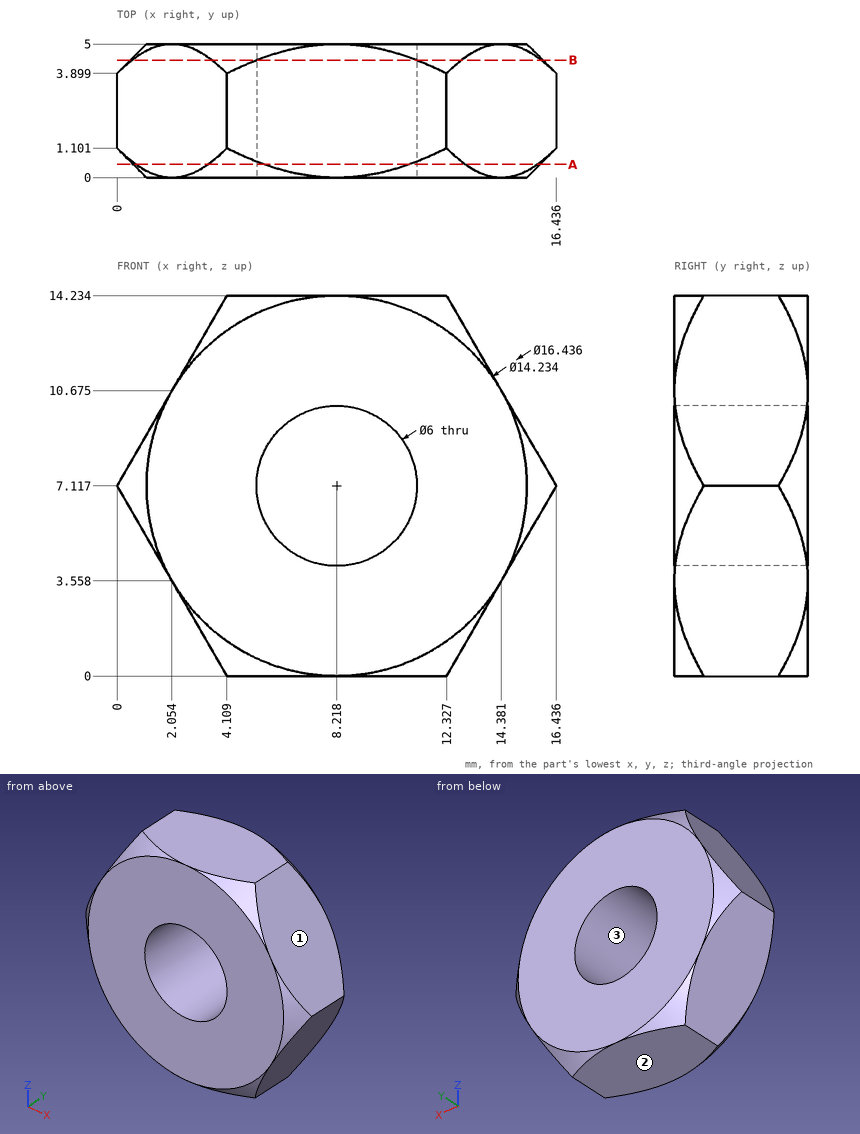
The figure shows three views and two pictorial views of one solid part (mm, origin at its lowest corner). Answer the questions. Give positions to 0.01 mm unless a question says otherwise; leave off trailing zeros. Order: outer loops, then holes, each group sorted by start corner. A loop starts at its lowest first (then second) coordinate and runs counter-clockwise, first axis right, second up. Notation, with made-up numbers: (36.5, 12) -> (53.5, 12) arc R11 ccw to (53.5, 27) -> close; hole circle Ø9 at (-17, 71.5). An arc over 180 degrees is marked (long way). Answer as a JSON object with one key per item and string values. Group by question number.
Item 1: Flat-ended cylindrical pins translate along their axes: pin 1 (1 mm diameter, centred on y = 4, z = 6, fed in from -X) (1 decimal); pin 2 (1.5 mm diameter, centred on y = 1, z = 12, fed in from -X) (1 decimal). Find the tip coordinate at first contact, or state that the pin passes through.
Item 2: Consider L1, parallel to X at y = 4.35, z = 8.25 (1 decimal); L2, parallel to Z at x = 6.75, y = 0.7 (1 decimal); L3, parallel to X at y = 2.35, z = 9.5 (1 decimal). Determine where each line is inside the solid, lowest interval first. Write a range as from..to.
Item 3: Determine the mould class of the marked faces 1, 2 and 3 for opening direction Z: pulls with the +Z half, pulls with the -Z half, needs draft (parallel to the pull), parting line crosses it, or undercut.
Item 4: The part is cut by section A-A on y = 0.5. Write down the section's boundary in (x, z) (1 decimal).
Item 5: The part is cut by section B-B on y = 4.4. Write down the section's boundary in (x, z) (1 decimal).
Result set:
{
 "1": {"pin 1": "x = 0.4", "pin 2": "x = 2.4"},
 "2": {"L1": "0.7..5.4, 11..15.8", "L2": "0..4.5, 9.7..14.2", "L3": "1.4..6.4, 10..15.1"},
 "3": {"face 1": "pulls with the +Z half", "face 2": "pulls with the -Z half", "face 3": "undercut"},
 "4": {"outline": "(0.7, 5.9) -> (3.4, 1.2) arc R7.6 ccw to (5.5, 0) -> (10.9, 0) arc R7.6 ccw to (13, 1.2) -> (15.7, 5.9) arc R7.6 ccw to (15.7, 8.3) -> (13, 13) arc R7.6 ccw to (10.9, 14.2) -> (5.5, 14.2) arc R7.6 ccw to (3.4, 13) -> (0.7, 8.3) arc R7.6 ccw to start; hole circle Ø6 at (8.2, 7.1)"},
 "5": {"outline": "(0.6, 6.1) -> (3.5, 1) arc R7.7 ccw to (5.2, 0) -> (11.2, 0) arc R7.7 ccw to (12.9, 1) -> (15.9, 6.1) arc R7.7 ccw to (15.9, 8.1) -> (12.9, 13.3) arc R7.7 ccw to (11.2, 14.2) -> (5.2, 14.2) arc R7.7 ccw to (3.5, 13.3) -> (0.6, 8.1) arc R7.7 ccw to start; hole circle Ø6 at (8.2, 7.1)"}
}
